Could you check a few things on this model? Use its own coordinates, in mm. Coordinates: 2 decimals unless noted, no trailing zeros. Order: outer loops, then holes, each group sorted by start corner. A loop starts at its lowest first (then second) coordinate and runs counter-clockwise, first axis right, second up. Notation, with made-up numbers: (-15, -19) - (8, -19) arc R28 cw to (8, 16) - close; hole circle Ø3 at (13.25, -38). An arc over 180 degrees is marked (long way). Answer as a JSON object with one key per item and string values. Group by question number.
(1) Imagine slicing it at B-B, the plane x = -39. Write out the boundary of the cut face in (y, z), and give its area (3 significant figures).
(2) Please list where these lines run through material, in increasing order: probe 1 along X at (y, z) = (2, 22.5); probe 2 along Z at (x, y) = (-46.5, 2); probe 3 along Z at (x, y) = (-20.5, 1).
(3) Imagine slicing it at A-A, the plane z = 55. Write out the boundary of the cut face in (x, y), and give its area (3 significant figures).
(4) Imagine slicing it at C-C, the plane y = 2.25. Give the number of separate pieces and of enclosed holes in the cut face, and give its area (3 significant figures).
from build123d import *

# Parameters (mm, degrees)
SKETCH1_W           = 160
SKETCH1_H           = 210
BOSS_EXTRUDE1_DEPTH = 8
SKETCH2_R           = 1.7
CUT_EXTRUDE1_DEPTH  = 37
FILLET1_R           = 10
SKETCH3_R           = 1.7
CUT_EXTRUDE2_DEPTH  = 480
SKETCH4_R           = 1.7
CUT_EXTRUDE3_DEPTH  = 480
SKETCH5_R           = 1.7
CUT_EXTRUDE4_DEPTH  = 480
FILLET2_R           = 1
CUT_EXTRUDE5_DEPTH  = 63


with BuildPart() as part:
    # Sketch1 → Boss-Extrude1 (new body)
    with BuildSketch(Plane(origin=(0, 0, 0), x_dir=(1, 0, 0), z_dir=(0, 1, 0))):
        Rectangle(SKETCH1_W, SKETCH1_H)
    extrude(amount=BOSS_EXTRUDE1_DEPTH)

    # Sketch2 → Cut-Extrude1 (cut)
    with BuildSketch(Plane(origin=(0, 8, 0), x_dir=(1, 0, 0), z_dir=(0, 1, 0))):
        with Locations(Location((-75, 22.5, 0), (0, 0, 270))):
            Circle(SKETCH2_R)
        with Locations(Location((-75, -22.5, 0), (0, 0, 270))):
            Circle(SKETCH2_R)
        with Locations(Location((75, 22.5, 0), (0, 0, 270))):
            Circle(SKETCH2_R)
        with Locations(Location((75, -22.5, 0), (0, 0, 270))):
            Circle(SKETCH2_R)
    extrude(amount=-CUT_EXTRUDE1_DEPTH, mode=Mode.SUBTRACT)

    # Fillet1
    fillet1_edges = [part.edges().sort_by_distance(p)[0] for p in [
        (80, 4, 105),
        (-80, 4, 105),
        (-80, 4, -105),
        (80, 4, -105),
    ]]
    fillet(fillet1_edges, radius=FILLET1_R)

    # Sketch3 → Cut-Extrude2 (cut)
    with BuildSketch(Plane(origin=(0, 8, 0), x_dir=(1, 0, 0), z_dir=(0, 1, 0))):
        with Locations(Location((-20, 22.5, 0), (0, 0, 270))):
            Circle(SKETCH3_R)
        with Locations(Location((-20, -22.5, 0), (0, 0, 270))):
            Circle(SKETCH3_R)
        with Locations(Location((20, -22.5, 0), (0, 0, 270))):
            Circle(SKETCH3_R)
        with Locations(Location((20, 22.5, 0), (0, 0, 270))):
            Circle(SKETCH3_R)
    extrude(amount=-CUT_EXTRUDE2_DEPTH, mode=Mode.SUBTRACT)

    # Sketch4 → Cut-Extrude3 (cut)
    with BuildSketch(Plane(origin=(0, 8, 0), x_dir=(1, 0, 0), z_dir=(0, 1, 0))):
        with Locations(Location((-75.005871396, 85, 0), (0, 0, 270))):
            Circle(SKETCH4_R)
        with Locations(Location((-60.011742792, 100, 0), (0, 0, 270))):
            Circle(SKETCH4_R)
        with Locations(Location((-75.005871396, -85, 0), (0, 0, 270))):
            Circle(SKETCH4_R)
        with Locations(Location((-60.011742792, -100, 0), (0, 0, 270))):
            Circle(SKETCH4_R)
        with Locations(Location((60.011742792, -100, 0), (0, 0, 270))):
            Circle(SKETCH4_R)
        with Locations(Location((75.005871396, -85, 0), (0, 0, 270))):
            Circle(SKETCH4_R)
        with Locations(Location((75.005871396, 85, 0), (0, 0, 270))):
            Circle(SKETCH4_R)
        with Locations(Location((60.011742792, 100, 0), (0, 0, 270))):
            Circle(SKETCH4_R)
    extrude(amount=-CUT_EXTRUDE3_DEPTH, mode=Mode.SUBTRACT)

    # Sketch5 → Cut-Extrude4 (cut)
    with BuildSketch(Plane(origin=(0, 8, 0), x_dir=(1, 0, 0), z_dir=(0, 1, 0))):
        with Locations(Location((35, -100, 0), (0, 0, 270))):
            Circle(SKETCH5_R)
        with Locations(Location((-35, -100, 0), (0, 0, 270))):
            Circle(SKETCH5_R)
        with Locations(Location((35, 100, 0), (0, 0, 270))):
            Circle(SKETCH5_R)
        with Locations(Location((-35, 100, 0), (0, 0, 270))):
            Circle(SKETCH5_R)
    extrude(amount=-CUT_EXTRUDE4_DEPTH, mode=Mode.SUBTRACT)

    # Fillet2
    fillet2_edges = [part.edges().sort_by_distance(p)[0] for p in [
        (0, 0, 105),
        (0, 8, 105),
        (80, 0, 0),
        (-80, 0, 0),
        (0, 0, -105),
        (-77.071067812, 0, -102.071067812),
        (77.071067812, 0, -102.071067812),
        (77.071067812, 0, 102.071067812),
        (-77.071067812, 0, 102.071067812),
        (-80, 8, 0),
        (80, 8, 0),
        (0, 8, -105),
        (-77.071067812, 8, -102.071067812),
        (77.071067812, 8, -102.071067812),
        (77.071067812, 8, 102.071067812),
        (-77.071067812, 8, 102.071067812),
    ]]
    fillet(fillet2_edges, radius=FILLET2_R)

    # Sketch6 → Cut-Extrude5 (cut)
    with BuildSketch(Plane(origin=(0, 8, 0), x_dir=(1, 0, 0), z_dir=(0, 1, 0))):
        with BuildLine():
            ThreePointArc((53.535533906, 36.464466094), (53.535533906, 73.535533906), (16.464466094, 73.535533906))
            ThreePointArc((16.464466094, 73.535533906), (16.464466094, 66.464466094), (23.535533906, 66.464466094))
            ThreePointArc((23.535533906, 66.464466094), (46.464466094, 66.464466094), (46.464466094, 43.535533906))
            ThreePointArc((46.464466094, 43.535533906), (46.464466094, 36.464466094), (53.535533906, 36.464466094))
        make_face()
        with BuildLine():
            ThreePointArc((-53.535533906, 36.464466094), (-53.535533906, 73.535533906), (-16.464466094, 73.535533906))
            ThreePointArc((-16.464466094, 73.535533906), (-16.464466094, 66.464466094), (-23.535533906, 66.464466094))
            ThreePointArc((-23.535533906, 66.464466094), (-46.464466094, 66.464466094), (-46.464466094, 43.535533906))
            ThreePointArc((-46.464466094, 43.535533906), (-46.464466094, 36.464466094), (-53.535533906, 36.464466094))
        make_face()
        with BuildLine():
            ThreePointArc((53.535533906, -36.464466094), (53.535533906, -73.535533906), (16.464466094, -73.535533906))
            ThreePointArc((16.464466094, -73.535533906), (16.464466094, -66.464466094), (23.535533906, -66.464466094))
            ThreePointArc((23.535533906, -66.464466094), (46.464466094, -66.464466094), (46.464466094, -43.535533906))
            ThreePointArc((46.464466094, -43.535533906), (46.464466094, -36.464466094), (53.535533906, -36.464466094))
        make_face()
        with BuildLine():
            ThreePointArc((-53.535533906, -36.464466094), (-53.535533906, -73.535533906), (-16.464466094, -73.535533906))
            ThreePointArc((-16.464466094, -73.535533906), (-16.464466094, -66.464466094), (-23.535533906, -66.464466094))
            ThreePointArc((-23.535533906, -66.464466094), (-46.464466094, -66.464466094), (-46.464466094, -43.535533906))
            ThreePointArc((-46.464466094, -43.535533906), (-46.464466094, -36.464466094), (-53.535533906, -36.464466094))
        make_face()
    extrude(amount=-CUT_EXTRUDE5_DEPTH, mode=Mode.SUBTRACT)


solid = part.part
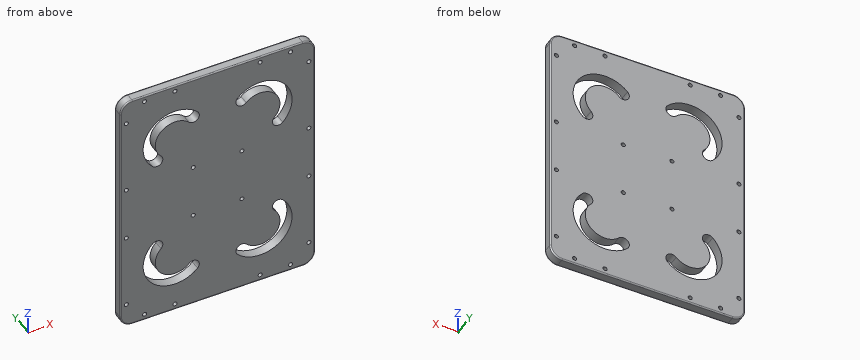
Result set:
{
 "1": {"outline": "(0, -104) arc R1 ccw to (1, -105) - (7, -105) arc R1 ccw to (8, -104) - (8, -80.91) - (0, -80.91) - close; (0, -70.71) - (8, -70.71) - (8, 70.71) - (0, 70.71) - close; (0, 80.91) - (8, 80.91) - (8, 104) arc R1 ccw to (7, 105) - (1, 105) arc R1 ccw to (0, 104) - close", "area": "1,520 mm^2"},
 "2": {"probe 1": "x = -80 to -76.7, -73.3 to -21.7, -18.3 to 18.3, 21.7 to 73.3, 76.7 to 80", "probe 2": "z = -105 to -78.56, -66.43 to -43.57, -36.43 to 36.43, 43.57 to 66.43, 78.56 to 105", "probe 3": "z = -105 to -76.84, -65.03 to -24.12, -20.88 to 20.88, 24.12 to 65.03, 76.84 to 105"},
 "3": {"outline": "(-80, 1) arc R1 ccw to (-79, 0) - (-61.21, 0) - (-61.21, 8) - (-79, 8) arc R1 ccw to (-80, 7) - close; (-51.21, 0) - (51.21, 0) - (51.21, 8) - (-51.21, 8) - close; (61.21, 0) - (79, 0) arc R1 ccw to (80, 1) - (80, 7) arc R1 ccw to (79, 8) - (61.21, 8) - close", "area": "1,120 mm^2"},
 "4": {"separate pieces": "1", "enclosed holes": "24", "area": "30,400 mm^2"}
}
